Geometry: see drawing. Coordinates: mm, zero at the bounding-box minimum. Round coordinates to 2 decimals unless told otherwise and drop trailing zeros. Loops run counter-clockwise (first coordinate to the right, second up) from the corner with the lowest first, then second, coordinate; pieces in that order, holes last.
(1) Section A-A, the plane z = 55. Return the cut outline in (x, y), plus the area to 3 significant figures.
(2) Section C-C, the plane y = 102. Return the cut outline in (x, z).
(3) First-contact query: pin 1 Ø8 at (x, z) = (11, 23.5) entering from -Y; pin 2 Ø5 at (x, y) = (61.5, 48) entering from +Z; pin 3 Ø3 at (x, y) = (91.5, 48) entering from -Z. Flat tips, straight axial feed; report the tip coordinate or a pass-through.
(4) Mould query, pull axis X, two halves, no side actions, for the marked faces 1, 2 and 3. Classes: pulls with the +X half, pulls with the -X half, needs draft (parallel to the pull), parting line crosses it, or undercut.
(5) Section B-B, the plane x = 55. Return the cut outline in (y, z), plus the area to 3 significant figures.
(6) Section D-D, the plane z = 97. Return the cut outline in (x, y).
(7) Material intervals for probe 1 along Z at (x, y) = (55, 57.5); probe 2 along Y at (x, z) = (96, 42), sorted ascending.
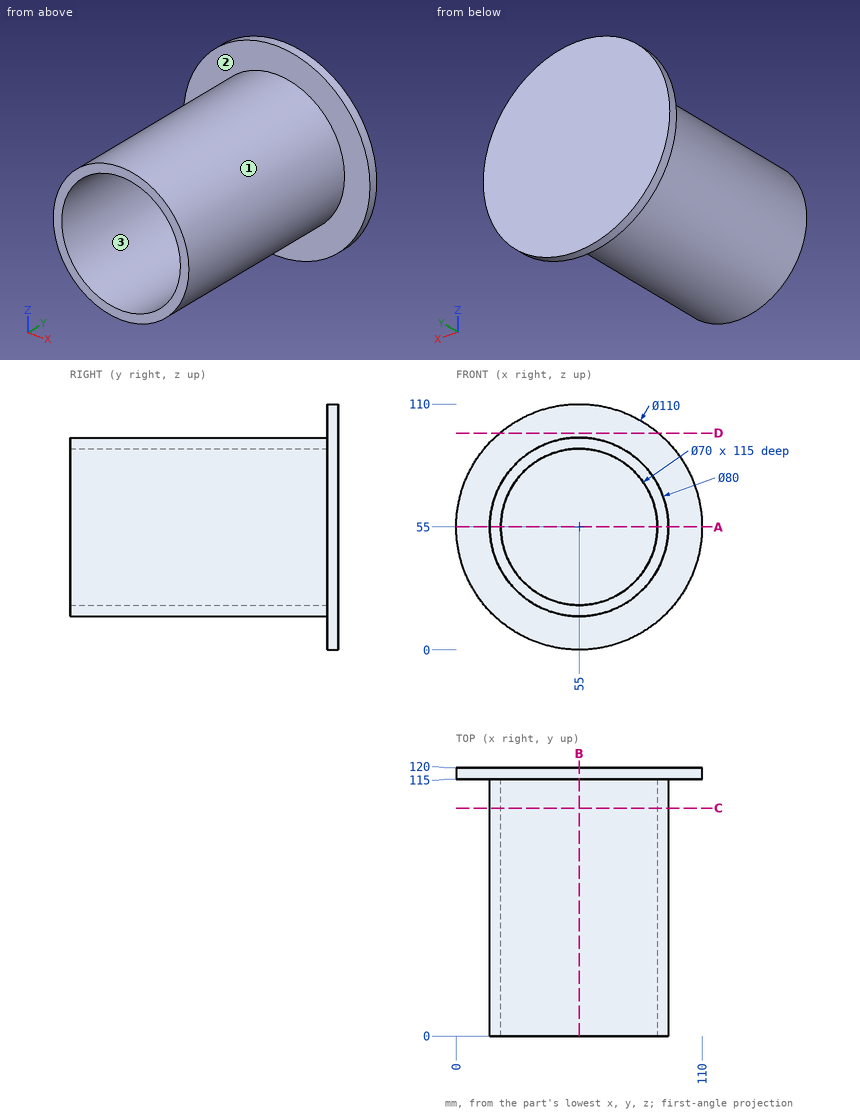
Output values:
1. outline: (0, 115) - (15, 115) - (15, 0) - (20, 0) - (20, 115) - (90, 115) - (90, 0) - (95, 0) - (95, 115) - (110, 115) - (110, 120) - (0, 120) - close
1. area: 1,700 mm2
2. outline: circle Ø80 at (55, 55); hole circle Ø70 at (55, 55)
3. pin 1: stops at y = 115
3. pin 2: stops at z = 94.8
3. pin 3: stops at z = 35.64
4. face 1: parting line crosses it
4. face 2: needs draft
4. face 3: undercut
5. outline: (0, 15) - (115, 15) - (115, 0) - (120, 0) - (120, 110) - (115, 110) - (115, 95) - (0, 95) - (0, 90) - (115, 90) - (115, 20) - (0, 20) - close
5. area: 1,700 mm2
6. outline: (19.49, 115) - (90.51, 115) - (90.51, 120) - (19.49, 120) - close
7. probe 1: z = 15 to 20, 90 to 95
7. probe 2: y = 115 to 120
